Geometry: final body of the model. Coordinates: model frame, mm. A direction names the side the tool comes from. Give positions to 0.01 mm unless a question says otherwise; leave off trailing zeros. Loops run counter-clockwise (first coordinate to the right, second up) from the corner with the lowest first, then second, coordinate; pieces in that order, holes last. Notation, with made-up numbers: (48, 74.5) -> (89, 74.5) arc R22 ccw to (89, 105.5) -> close; hole circle Ø1 at (64.25, 85). An arc over 180 degrees is marked (long way). One line per question, with ' | ' between items. Start each with the question number.
Item 1: Section B-B on z = 22. Return loops of the section in (x, y), then the cut area to 3 significant figures.
Item 2: Material intervals for line 1 along Y through (x, z) = (-24, 3); line 2 along X through (y, z) = (34, 13); line 3 along Z through (x, y) = (-4, 25.5), sorted ascending. Write a range as [from, to].
Item 3: Section A-A on y = 17.5. Return loops of the section in (x, z).
Item 4: Set-up query: faces 1 (the flat face through (-28, 20, 15)), 2 (the cylindrical face through (-10.14, 34.297, 13.986)), 3 (the flat face through (-10, 10, 30)). Return all of +Z, -Z, +X, -X, +Y, -Y with unobstructed straight access to the full face (end or side cutting, diameter ignored); none if empty.
Item 5: Pin query (flat end, axial travel): P1, Ø16, axis at x = -28, z = 23.5, coming from the +Y side; P2, Ø16, axis at y = 28.5, z = 5.5, coming from the -X side; P3, Ø5, axis at y = 29.5, z = 21, coming from the -X side; P4, Ø10, axis at x = -16.5, y = 28.5, coming from the +Z side. Return the tip coordinate at first contact, or that it passes through.
Item 6: Section D-D on x = -36. Return loops of the section in (y, z), then the cut area to 3 significant figures.
Item 7: Section C-C on x = -29. Return loops of the section in (y, z), then the cut area to 3 significant figures.
from build123d import *

# Parameters (mm, degrees)
BOSS_EXTRUDE1_DEPTH = 40
CUT_EXTRUDE1_DEPTH  = 40
CUT_EXTRUDE2_DEPTH  = 40
CUT_EXTRUDE4_DEPTH  = 20


with BuildPart() as part:
    # Sketch1 → Boss-Extrude1 (new body)
    with BuildSketch(Plane.XY):
        Polygon((0, 0), (0, 40), (-20, 40), (-20, 20), (-40, 20), (-40, 0), align=None)
    extrude(amount=BOSS_EXTRUDE1_DEPTH)

    # Sketch3 → Cut-Extrude1 (cut)
    with BuildSketch(Plane.ZY.offset(20)):
        with BuildLine():
            Line((40, 40), (0, 40))
            ThreePointArc((0, 40), (14.142135624, 34.142135624), (20, 20))
            Line((20, 20), (40, 20))
            Line((40, 20), (40, 40))
        make_face()
    extrude(amount=-CUT_EXTRUDE1_DEPTH, mode=Mode.SUBTRACT)

    # Sketch5 → Cut-Extrude2 (cut)
    with BuildSketch(Plane(origin=(0, 20, 0), x_dir=(1, 0, 0), z_dir=(0, 1, 0))):
        Polygon((-20, -40), (-40, -10), (-40, -40), align=None)
    extrude(amount=-CUT_EXTRUDE2_DEPTH, mode=Mode.SUBTRACT)

    # Sketch8 → Cut-Extrude4 (cut)
    with BuildSketch(Plane(origin=(0, 0, 0), x_dir=(0, 0, -1), z_dir=(1, 0, 0))):
        Polygon((-20, 20), (-40, 0), (-40, 20), align=None)
    extrude(amount=-CUT_EXTRUDE4_DEPTH, mode=Mode.SUBTRACT)


solid = part.part
Result sheet:
1) outline: (-32, 0) -> (0, 0) -> (0, 18) -> (-20, 18) -> (-20, 20) -> (-32, 20) -> close | area: 600 mm²
2) line 1: y = [0, 20] | line 2: x = [-20, 0] | line 3: z = [0, 19.23]
3) outline: (-40, 0) -> (0, 0) -> (0, 22.5) -> (-20, 22.5) -> (-20, 40) -> (-40, 10) -> close
4) face 1: +Z, -Z, -X, +Y | face 2: +Z, +X, -X, +Y | face 3: +Z, +X, +Y
5) P1: stops at y = 20 | P2: stops at x = -20 | P3: passes through | P4: stops at z = 19.69
6) outline: (0, 0) -> (20, 0) -> (20, 16) -> (0, 16) -> close | area: 320 mm²
7) outline: (0, 0) -> (20, 0) -> (20, 26.5) -> (0, 26.5) -> close | area: 530 mm²
